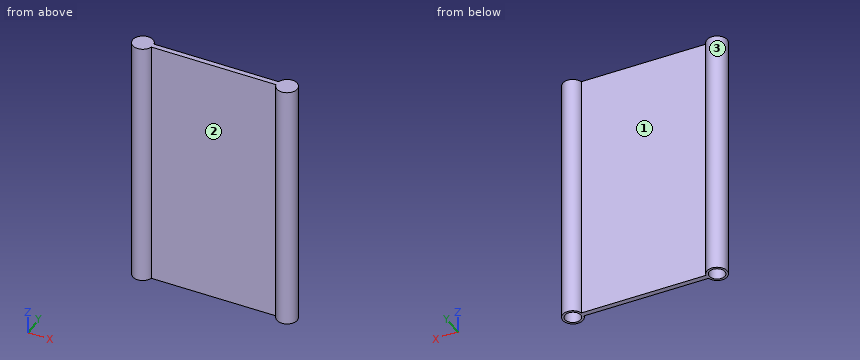
Autodesk Fusion 360 part; units mm, degrees
sketch "Sketch1" plane through (0, 0, 0) normal (0, 0, 1) x (1, 0, 0)
  circle A0 centre (0, 0) radius 3
  dimension "d1" = 6
extrude "Extrude1" add sketch "Sketch1" along normal blind 100
thread "Thread1" thread offset 0 thread length 10

Autodesk Fusion 360 part; units mm, degrees
sketch "Sketch1" plane through (0, 0, 0) normal (0, 0, 1) x (1, 0, 0)
  circle A0 centre (-28.5, 0) radius 4
  circle A1 centre (28.5, 0) radius 4
  line L0 (-24.627, 1) -> (24.627, 1)
  line L1 (-24.627, -1) -> (24.627, -1)
  dimension "d1" = 8
  dimension "d2" = 28.5
  dimension "d3" = 8
  dimension "d4" = 28.5
  dimension "d5" = 1
  dimension "d6" = 1
extrude "Extrude1" add sketch "Sketch1" along normal blind 80
sketch "Sketch2" plane through (0, 0, 80) normal (0, 0, 1) x (-1, 0, 0)
  arc A0 (24.627, -1) -> (24.627, 1) centre (28.5, 0) ccw
  line L0 (24.627, 1) -> (-24.627, 1)
  arc A1 (-24.627, 1) -> (-24.627, -1) centre (-28.5, 0) ccw
  line L1 (-24.627, -1) -> (24.627, -1)
  circle A2 centre (28.5, 0) radius 3.1
  circle A3 centre (-28.5, 0) radius 3.1
  dimension "d9" = 6.2
  dimension "d10" = 6.2
extrude "Extrude2" cut sketch "Sketch2" against normal blind 90 contours A2 | A3
thread "Thread1" thread offset 0 thread length 10
thread "Thread2" thread offset 0 thread length 10
Geometry: final body of the model. Coordinates: model frame, mm. Face numbers are marked on the shaded views. A direction names the side the tool comes from. Round coordinates to 2 decimals unless told otherwise and drop trailing zeros. Write each loop counter-clockwise with the first axis right and the second up, starting at its lowest first coordinate (ties: lowest second). Pieces come first, ordered by that corner, then holes. Notation, with made-up numbers: M 81.25,12 L 97.25,12 A13 cw 97.25,37 Z; hole C 30.5,69.5 d2. An arc over 180 degrees is marked long. Answer in a Markdown table with one row per item. Add a question column.
(1) Cut plane D-D, the plane x = -12. Return the cut outline in (y, z).
(2) Cut plane C-C, the plane z = 6. Return the cut outline in (x, y), then the cut area to 3 significant figures.
(3) Contact query for flat-ended pins moving along their axis: pin 1 (24.5 mm diameter, centred on x = -2, z = 42.5, fed in from -Y); pin 2 (2 mm diameter, centred on y = 1, z = 30.5, fed in from -X); pin 3 (1.9 mm diameter, centred on x = -29, y = 0, fed in from -Z); pin 4 (1.5 mm diameter, centred on x = -13, z = 39, fed in from +Y). Output: stop coordinate, or through.
(4) Cut plane B-B, the plane x = 28.5. Return the cut outline in (y, z).
(5) Ray query, L1, parallel to X at y = 0, z = 58; L2, parallel to Y at x = 28.5, z = 63.5; L3, parallel to X at y = 1.75, z = 7.5. Return the intervals inside material, ascending.
(6) Cut plane A-A, the plane y = 0. Return the cut outline in (x, z).
(7) Reachability of the marked faces 1, 2 and 3 from +Z, -Z, +X, -X, +Y, -Y: full face, straight path, thin tool, end or side. Return the list, or none.
Established:
| question | item | result |
|---|---|---|
| 1 | outline | M -1,0 L 1,0 L 1,100 L -1,100 Z |
| 2 | outline | M -24.63,-1 L 24.63,-1 A4 ccw long 24.63,1 L -24.63,1 A4 ccw long Z; hole C -28.5,0 d6.2; hole C 28.5,0 d6.2 |
| 2 | area | 138 mm² |
| 3 | pin 1 | y = -1 |
| 3 | pin 2 | x = -32.5 |
| 3 | pin 3 | z = 80 |
| 3 | pin 4 | y = 1 |
| 4 | outline | M -4,0 L -3.1,0 L -3.1,80 L 3.1,80 L 3.1,0 L 4,0 L 4,100 L -4,100 Z |
| 5 | L1 | -32.5 to -31.6, -25.4 to 25.4, 31.6 to 32.5 |
| 5 | L2 | -4 to -3.1, 3.1 to 4 |
| 5 | L3 | -32.1 to -31.06, -25.94 to -24.9, 24.9 to 25.94, 31.06 to 32.1 |
| 6 | outline | M -32.5,0 L -31.6,0 L -31.6,80 L -25.4,80 L -25.4,0 L 25.4,0 L 25.4,80 L 31.6,80 L 31.6,0 L 32.5,0 L 32.5,100 L -32.5,100 Z |
| 7 | face 1 | +Z, -Z, +Y |
| 7 | face 2 | +Z, -Z, -Y |
| 7 | face 3 | +Z, -Z |
